Read the model definition and answer for the solid it produces. Units are mm, in the model's axes. A direction names the side the tool comes from. Coordinates: 2 decimals unless noted, no trailing zeros. Order: outer loops, then holes, each group sorted by start corner. A loop starts at its lowest first (then second) coordinate and runs counter-clockwise, first axis right, second up. Notation, with made-up numbers: (87.5, 76) - (103.5, 76) arc R26 ccw to (103.5, 100) - close; hole circle Ø9 at (77, 80). An arc over 180 degrees is marked (long way). Answer as a JSON object with one key per item and string values. Group by question number.
from build123d import *

# Parameters (mm, degrees)
SKETCH1_R                    = 2.5
BASE_FLANGE1_DEPTH           = 3
EDGE_FLANGE1_STRIP_W         = 13
EDGE_FLANGE1_STRIP_H         = 3
EDGE_FLANGE1_STRIP_CUT_DEPTH = 54
EDGE_FLANGE1_DEPTH           = 54
EDGE_FLANGE2_DEPTH           = 54
SKETCH25_R                   = 2.5
CUT_EXTRUDE1_DEPTH           = 65.67835805


# Sheet-metal steps are written as plain solids
with BuildPart() as part:
    # Sketch1 → Base-Flange1 (new body)
    with BuildSketch(Plane(origin=(0, 0, 0), x_dir=(1, 0, 0), z_dir=(0, 1, 0))):
        with BuildLine():
            Line((0, 0), (54, 0))
            Line((54, 0), (54, 11))
            ThreePointArc((54, 11), (52.535533906, 14.535533906), (49, 16))
            Line((49, 16), (5, 16))
            ThreePointArc((5, 16), (1.464466094, 14.535533906), (0, 11))
            Line((0, 11), (0, 0))
        make_face()
        with Locations(Location((8, 8, 0), (0, 0, 270))):
            Circle(SKETCH1_R, mode=Mode.SUBTRACT)
        with Locations(Location((46, 8, 0), (0, 0, 90))):
            Circle(SKETCH1_R, mode=Mode.SUBTRACT)
    extrude(amount=-BASE_FLANGE1_DEPTH)

    # Edge-Flange1 strip (across the edge) → Edge-Flange1 strip cut (cut)
    with BuildSketch(Plane(origin=(0, 0, 0), x_dir=(0, 0, -1), z_dir=(1, 0, 0))):
        with Locations((-6, -1.5)):
            Rectangle(EDGE_FLANGE1_STRIP_W, EDGE_FLANGE1_STRIP_H)
    extrude(amount=EDGE_FLANGE1_STRIP_CUT_DEPTH, mode=Mode.SUBTRACT)

    # Edge-Flange1 section (across the edge) → Edge-Flange1 (add)
    with BuildSketch(Plane(origin=(0, 0, 0), x_dir=(0, 0, -1), z_dir=(1, 0, 0))):
        with BuildLine():
            Line((-3, 0.5), (-3, 1))
            Line((-3, 1), (0, 1))
            Line((0, 1), (0, 0.5))
            ThreePointArc((0, 0.5), (0.146446609, 0.146446609), (0.5, 0))
            Line((0.5, 0), (0.5, -3))
            ThreePointArc((0.5, -3), (-1.974873734, -1.974873734), (-3, 0.5))
        make_face()
    extrude(amount=EDGE_FLANGE1_DEPTH)

    # Edge-Flange2 section (across the edge) → Edge-Flange2 (add)
    with BuildSketch(Plane(origin=(54, 1.5, 3), x_dir=(0, -1, 0), z_dir=(-1, 0, 0))):
        with BuildLine():
            Line((-3, 0.5), (-3, 31.8))
            Line((-3, 31.8), (0, 31.8))
            Line((0, 31.8), (0, 0.5))
            ThreePointArc((0, 0.5), (0.146446609, 0.146446609), (0.5, 0))
            Line((0.5, 0), (0.5, -3))
            ThreePointArc((0.5, -3), (-1.974873734, -1.974873734), (-3, 0.5))
        make_face()
    extrude(amount=EDGE_FLANGE2_DEPTH)

    # Sketch25 → Cut-Extrude1 (cut, through all)
    with BuildSketch(Plane(origin=(0, 4.5, 0), x_dir=(1, 0, 0), z_dir=(0, 1, 0))):
        with Locations(Location((27, -26.8, 0), (0, 0, 270))):
            Circle(SKETCH25_R)
        with Locations(Location((8, -26.8, 0), (0, 0, 270))):
            Circle(SKETCH25_R)
        with BuildLine():
            ThreePointArc((8, -34.8), (2.343145751, -32.456854249), (0, -26.8))
            Line((0, -26.8), (0, -34.8))
            Line((0, -34.8), (8, -34.8))
        make_face()
        with Locations(Location((46, -26.8, 0), (0, 0, 270))):
            Circle(SKETCH25_R)
        with BuildLine():
            Line((54, -34.8), (54, -26.8))
            ThreePointArc((54, -26.8), (51.656854249, -32.456854249), (46, -34.8))
            Line((46, -34.8), (54, -34.8))
        make_face()
    extrude(amount=-CUT_EXTRUDE1_DEPTH, mode=Mode.SUBTRACT)


solid = part.part
1. A cutting plane is placed at B-B on x = 27. Write down the section's boundary in (y, z).
2. A cutting plane is placed at D-D on y = -1.25. Write down the section's boundary in (x, z).
3. For faces 4 (the flat face through (27, 0, -8)), 5 (the flat face through (27, 1.5, 19)), 6 (the flat face through (54, 2, 8)), determine the directions among +Z, -Z, +X, -X, +Y, -Y from which every point of the face is accessible in a straight line to the end or side of a thin tool.
4. For a pull along Z with two mould halves and no side action, classify faces 1 (the cylindrical face through (27.38, 3.45, 1)), 2 (the cylindrical face through (43.56, 3.02, 26.26)), 3 (the flat face through (0, 2, 8)) as pulls with the +Z half, pulls with the -Z half, needs draft (parallel to the pull), parting line crosses it, or undercut.
5. A cutting plane is placed at C-C on z = 28.5. Write down the section's boundary in (x, y).
6. A cutting plane is placed at A-A on z = -8. Write down the section's boundary in (x, y), and give its area (3 significant figures).
7. Given pin 1 (12.5 mm diameter, centred on x = 28.5, z = -8, fed in from +Y); pin 2 (2 mm diameter, centred on y = 1, z = 11, fed in from -X), each flat-ended and moving along its own axis, determine where each tip first touches the part or whether it passes through.
8. Straight lines are drawn through the part: L1, parallel to X at y = -0.65, z = -8; L2, parallel to X at y = 3.9, z = 26.8; L3, parallel to X at y = 4, z = 28.5. For each, find the intervals that lie inside material, in ascending order.
Derived:
{
 "1": {"outline": "(-3, -16) - (0, -16) - (0, -0.5) arc R0.5 cw to (0.5, 0) - (1, 0) arc R3.5 ccw to (4.5, 3.5) - (4.5, 24.3) - (1.5, 24.3) - (1.5, 3.5) arc R0.5 cw to (1, 3) - (0.5, 3) arc R3.5 ccw to (-3, -0.5) - close; (1.5, 29.3) - (4.5, 29.3) - (4.5, 34.8) - (1.5, 34.8) - close"},
 "2": {"outline": "(0, -11) arc R5 ccw to (5, -16) - (49, -16) arc R5 ccw to (54, -11) - (54, 2.53) - (0, 2.53) - close; hole circle Ø5 at (8, -8); hole circle Ø5 at (46, -8)"},
 "3": {"face 4": "-Z, +X, -X, +Y", "face 5": "+Z, +X, -X, -Y", "face 6": "+Z, -Z, +X, +Y, -Y"},
 "4": {"face 1": "pulls with the -Z half", "face 2": "undercut", "face 3": "needs draft"},
 "5": {"outline": "(0.18, 1.5) - (6.17, 1.5) - (6.17, 4.5) - (0.18, 4.5) - close; (9.83, 1.5) - (25.17, 1.5) - (25.17, 4.5) - (9.83, 4.5) - close; (28.83, 1.5) - (44.17, 1.5) - (44.17, 4.5) - (28.83, 4.5) - close; (47.83, 1.5) - (53.82, 1.5) - (53.82, 4.5) - (47.83, 4.5) - close"},
 "6": {"outline": "(0, -3) - (5.5, -3) - (5.5, 0) - (0, 0) - close; (10.5, -3) - (43.5, -3) - (43.5, 0) - (10.5, 0) - close; (48.5, -3) - (54, -3) - (54, 0) - (48.5, 0) - close", "area": "132 mm2"},
 "7": {"pin 1": "stops at y = 0", "pin 2": "stops at x = 0"},
 "8": {"L1": "x = 0 to 5.5, 10.5 to 43.5, 48.5 to 54", "L2": "x = 0 to 5.5, 10.5 to 24.5, 29.5 to 43.5, 48.5 to 54", "L3": "x = 0.18 to 6.17, 9.83 to 25.17, 28.83 to 44.17, 47.83 to 53.82"}
}
